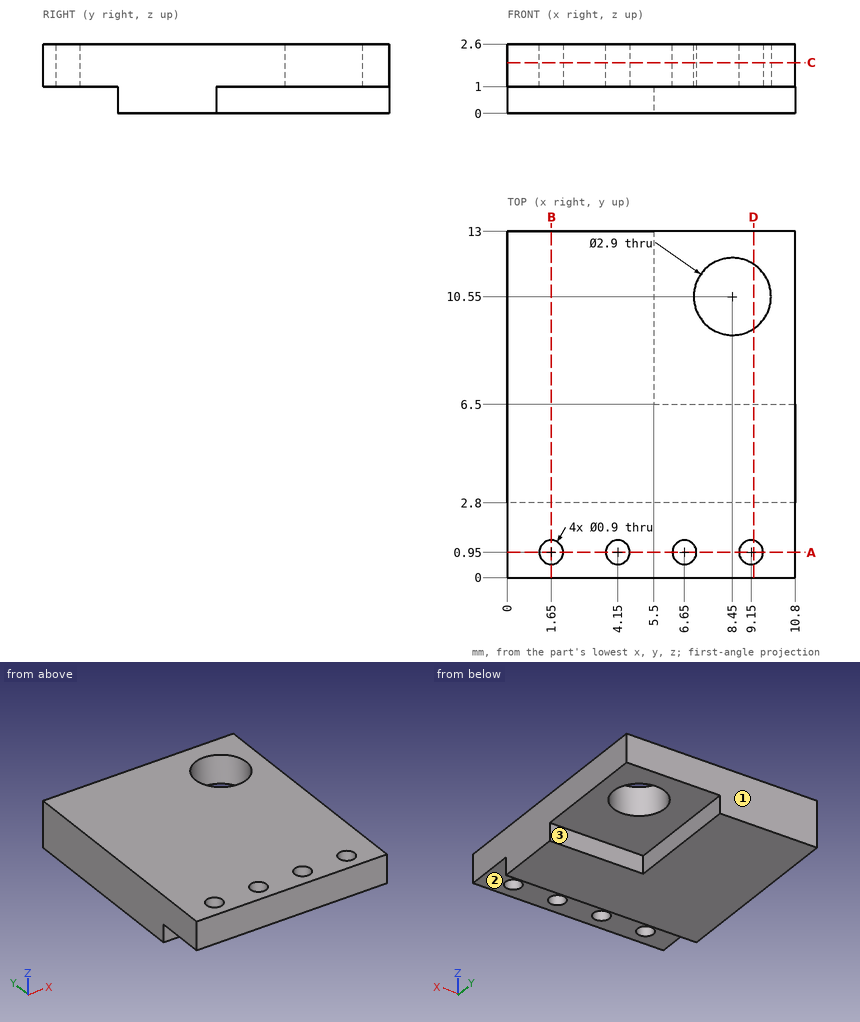
Input: dimensioned drawing with shaded views. Units: mm. Origin: part minimum x, y, z. A direction names the side the tool comes from. Coordinates: 2 decimals unless noted, no trailing zeros. Order: outer loops, then holes, each group sorted by start corner. A loop starts at its lowest first (then second) coordinate and runs counter-clockwise, first axis right, second up.
(1) Section query D-D (x = 9.25). Return the cut outline in (y, z).
(2) First-contact query: pin 1 (0.5 mm diameter, centred on x = 7.5, z = 0.5, fed in from +Y); pin 2 (1.7 mm diameter, centred on x = 8.45, y = 10.55, fed in from -Z); pin 3 (0.8 mm diameter, centred on x = 3.5, y = 1.5, fed in from -Z). Flat tips, straight axial feed; report the tip coordinate or a pass-through.
(3) Section query B-B (x = 1.65). Return the cut outline in (y, z), plus the area to 3 significant figures.
(4) Access query for the marked faces 1, 2 and 3. Directions: +Z, -Z, +X, -X, +Y, -Y. A direction counts if a zero-diameter tool reaches every point of the face in a straight line with its end or side. Return the directions, or none.
(5) Section query C-C (z = 1.9). Return the cut outline in (x, y), plus the area to 3 significant figures.
(6) Material intervals for probe 1 along Y at (x, z) = (4.15, 2.05); probe 2 along Y at (x, z) = (9.5, 2.1); probe 3 along Y at (x, z) = (9.25, 1.9), sorted ascending.
(7) Section query A-A (y = 0.95). Return the cut outline in (x, z), plus the area to 3 significant figures.
Solution:
1. outline: (0, 1) - (0.51, 1) - (0.51, 2.6) - (0, 2.6) - close; (1.39, 1) - (2.8, 1) - (2.8, 0) - (6.5, 0) - (6.5, 1) - (9.34, 1) - (9.34, 2.6) - (1.39, 2.6) - close; (11.76, 1) - (13, 1) - (13, 2.6) - (11.76, 2.6) - close
2. pin 1: stops at y = 6.5
2. pin 2: passes through
2. pin 3: stops at z = 1
3. outline: (0, 1) - (0.5, 1) - (0.5, 2.6) - (0, 2.6) - close; (1.4, 1) - (2.8, 1) - (2.8, 0) - (13, 0) - (13, 2.6) - (1.4, 2.6) - close
3. area: 29.6 mm2
4. face 1: +Z, -Z, +X, -X, +Y
4. face 2: -Z, +X, -X, -Y
4. face 3: -Z, +X, +Y
5. outline: (0, 0) - (10.8, 0) - (10.8, 13) - (0, 13) - close; hole circle Ø0.9 at (1.65, 0.95); hole circle Ø0.9 at (4.15, 0.95); hole circle Ø0.9 at (6.65, 0.95); hole circle Ø2.9 at (8.45, 10.55); hole circle Ø0.9 at (9.15, 0.95)
5. area: 131 mm2
6. probe 1: y = 0 to 0.5, 1.4 to 13
6. probe 2: y = 0 to 0.67, 1.23 to 9.55, 11.55 to 13
6. probe 3: y = 0 to 0.51, 1.39 to 9.34, 11.76 to 13
7. outline: (0, 1) - (1.2, 1) - (1.2, 2.6) - (0, 2.6) - close; (2.1, 1) - (3.7, 1) - (3.7, 2.6) - (2.1, 2.6) - close; (4.6, 1) - (6.2, 1) - (6.2, 2.6) - (4.6, 2.6) - close; (7.1, 1) - (8.7, 1) - (8.7, 2.6) - (7.1, 2.6) - close; (9.6, 1) - (10.8, 1) - (10.8, 2.6) - (9.6, 2.6) - close
7. area: 11.5 mm2
